```python
from build123d import *

# Parameters (mm, degrees)
SKETCH2_W            = 260
SKETCH2_H            = 260
BOSS_EXTRUDE1_DEPTH  = 500
SKETCH4_W            = 40
SKETCH4_H            = 60
CUT_EXTRUDE1_DEPTH   = 621.644825967
CUT_EXTRUDE2_REACH   = 622.645
MIRROR2_COPY_1_REACH = 622.645


with BuildPart() as part:
    # Sketch2 → Boss-Extrude1 (new body)
    with BuildSketch(Plane(origin=(0, 0, 0), x_dir=(1, 0, 0), z_dir=(0, 1, 0))):
        with Locations((130, 130)):
            Rectangle(SKETCH2_W, SKETCH2_H)
    extrude(amount=BOSS_EXTRUDE1_DEPTH)

    # Sketch4 → Cut-Extrude1 (cut, symmetric)
    with BuildSketch(Plane(origin=(260, 0, 0), x_dir=(0, 0, -1), z_dir=(1, 0, 0))):
        with Locations((20, 370)):
            Rectangle(SKETCH4_W, SKETCH4_H)
    cut_extrude1 = extrude(amount=CUT_EXTRUDE1_DEPTH, both=True, mode=Mode.SUBTRACT)

    # Sketch5 → Cut-Extrude2 (cut, up to next)
    with BuildSketch(Plane(origin=(0, 500, 0), x_dir=(1, 0, 0), z_dir=(0, 1, 0)), mode=Mode.PRIVATE) as cut_extrude2_sk1:
        with BuildLine():
            ThreePointArc((69.556138468, 20.047965883), (67.212992718, 25.704820132), (61.556138468, 28.047965883))
            Line((61.556138468, 28.047965883), (61.556138468, 20.047965883))
            Line((61.556138468, 20.047965883), (61.556138468, 12.047965883))
            ThreePointArc((61.556138468, 12.047965883), (67.212992718, 14.391111633), (69.556138468, 20.047965883))
        make_face()
    cut_extrude2_tool1 = extrude(cut_extrude2_sk1.sketch, amount=-CUT_EXTRUDE2_REACH, mode=Mode.PRIVATE) & part.part
    # Sketch5 → Cut-Extrude2 (cut, up to next)
    with BuildSketch(Plane(origin=(0, 500, 0), x_dir=(1, 0, 0), z_dir=(0, 1, 0)), mode=Mode.PRIVATE) as cut_extrude2_sk2:
        with BuildLine():
            Line((61.556138468, 20.047965883), (61.556138468, 28.047965883))
            ThreePointArc((61.556138468, 28.047965883), (53.556138468, 20.047965883), (61.556138468, 12.047965883))
            Line((61.556138468, 12.047965883), (61.556138468, 20.047965883))
        make_face()
    cut_extrude2_tool2 = extrude(cut_extrude2_sk2.sketch, amount=-CUT_EXTRUDE2_REACH, mode=Mode.PRIVATE) & part.part
    # Sketch5 → Cut-Extrude2 (cut, up to next)
    with BuildSketch(Plane(origin=(0, 500, 0), x_dir=(1, 0, 0), z_dir=(0, 1, 0)), mode=Mode.PRIVATE) as cut_extrude2_sk3:
        with BuildLine():
            ThreePointArc((69.556138468, 20.047965883), (67.212992718, 25.704820132), (61.556138468, 28.047965883))
            Line((61.556138468, 28.047965883), (61.556138468, 20.047965883))
            Line((61.556138468, 20.047965883), (61.556138468, 12.047965883))
            ThreePointArc((61.556138468, 12.047965883), (67.212992718, 14.391111633), (69.556138468, 20.047965883))
        make_face()
    cut_extrude2_tool3 = extrude(cut_extrude2_sk3.sketch, amount=-CUT_EXTRUDE2_REACH, mode=Mode.PRIVATE) & part.part
    # Sketch5 → Cut-Extrude2 (cut, up to next)
    with BuildSketch(Plane(origin=(0, 500, 0), x_dir=(1, 0, 0), z_dir=(0, 1, 0)), mode=Mode.PRIVATE) as cut_extrude2_sk4:
        with BuildLine():
            Line((61.556138468, 20.047965883), (61.556138468, 28.047965883))
            ThreePointArc((61.556138468, 28.047965883), (53.556138468, 20.047965883), (61.556138468, 12.047965883))
            Line((61.556138468, 12.047965883), (61.556138468, 20.047965883))
        make_face()
    cut_extrude2_tool4 = extrude(cut_extrude2_sk4.sketch, amount=-CUT_EXTRUDE2_REACH, mode=Mode.PRIVATE) & part.part
    cut_extrude2_1 = cut_extrude2_tool1.solids().sort_by_distance((64.951444, 500, -20.047966))[0]
    add(cut_extrude2_1, mode=Mode.SUBTRACT)
    cut_extrude2_2 = cut_extrude2_tool2.solids().sort_by_distance((58.160833, 500, -20.047966))[0]
    add(cut_extrude2_2, mode=Mode.SUBTRACT)
    cut_extrude2_3 = cut_extrude2_tool3.solids().sort_by_distance((64.951444, 500, -20.047966))[0]
    add(cut_extrude2_3, mode=Mode.SUBTRACT)
    cut_extrude2_4 = cut_extrude2_tool4.solids().sort_by_distance((58.160833, 500, -20.047966))[0]
    add(cut_extrude2_4, mode=Mode.SUBTRACT)
    cut_extrude2 = cut_extrude2_1 + cut_extrude2_2 + cut_extrude2_3 + cut_extrude2_4  # Cut-Extrude2 as one shape, for the pattern or mirror that repeats it

    # Mirror1: Cut-Extrude2 across plane
    add(cut_extrude2.mirror(Plane.ZY.offset(-130)), mode=Mode.SUBTRACT)

    # Mirror2: Cut-Extrude1, Cut-Extrude2 across plane
    add(cut_extrude1.mirror(Plane(origin=(0, 0, -130), x_dir=(1, 0, 0), z_dir=(0, 0, -1))), mode=Mode.SUBTRACT)
    add(cut_extrude2.mirror(Plane(origin=(0, 0, -130), x_dir=(1, 0, 0), z_dir=(0, 0, -1))), mode=Mode.SUBTRACT)

    # Mirror2 copy 1 sketch → Mirror2 copy 1 (cut, up to next)
    with BuildSketch(Plane(origin=(260, 500, -260), x_dir=(-1, 0, 0), z_dir=(0, 1, 0)), mode=Mode.PRIVATE) as mirror2_copy_1_sk1:
        with BuildLine():
            ThreePointArc((69.556138468, 20.047965883), (67.212992718, 25.704820132), (61.556138468, 28.047965883))
            Line((61.556138468, 28.047965883), (61.556138468, 20.047965883))
            Line((61.556138468, 20.047965883), (61.556138468, 12.047965883))
            ThreePointArc((61.556138468, 12.047965883), (67.212992718, 14.391111633), (69.556138468, 20.047965883))
        make_face()
    mirror2_copy_1_tool1 = extrude(mirror2_copy_1_sk1.sketch, amount=-MIRROR2_COPY_1_REACH, mode=Mode.PRIVATE) & part.part
    # Mirror2 copy 1 sketch → Mirror2 copy 1 (cut, up to next)
    with BuildSketch(Plane(origin=(260, 500, -260), x_dir=(-1, 0, 0), z_dir=(0, 1, 0)), mode=Mode.PRIVATE) as mirror2_copy_1_sk2:
        with BuildLine():
            Line((61.556138468, 20.047965883), (61.556138468, 28.047965883))
            ThreePointArc((61.556138468, 28.047965883), (53.556138468, 20.047965883), (61.556138468, 12.047965883))
            Line((61.556138468, 12.047965883), (61.556138468, 20.047965883))
        make_face()
    mirror2_copy_1_tool2 = extrude(mirror2_copy_1_sk2.sketch, amount=-MIRROR2_COPY_1_REACH, mode=Mode.PRIVATE) & part.part
    # Mirror2 copy 1 sketch → Mirror2 copy 1 (cut, up to next)
    with BuildSketch(Plane(origin=(260, 500, -260), x_dir=(-1, 0, 0), z_dir=(0, 1, 0)), mode=Mode.PRIVATE) as mirror2_copy_1_sk3:
        with BuildLine():
            ThreePointArc((69.556138468, 20.047965883), (67.212992718, 25.704820132), (61.556138468, 28.047965883))
            Line((61.556138468, 28.047965883), (61.556138468, 20.047965883))
            Line((61.556138468, 20.047965883), (61.556138468, 12.047965883))
            ThreePointArc((61.556138468, 12.047965883), (67.212992718, 14.391111633), (69.556138468, 20.047965883))
        make_face()
    mirror2_copy_1_tool3 = extrude(mirror2_copy_1_sk3.sketch, amount=-MIRROR2_COPY_1_REACH, mode=Mode.PRIVATE) & part.part
    # Mirror2 copy 1 sketch → Mirror2 copy 1 (cut, up to next)
    with BuildSketch(Plane(origin=(260, 500, -260), x_dir=(-1, 0, 0), z_dir=(0, 1, 0)), mode=Mode.PRIVATE) as mirror2_copy_1_sk4:
        with BuildLine():
            Line((61.556138468, 20.047965883), (61.556138468, 28.047965883))
            ThreePointArc((61.556138468, 28.047965883), (53.556138468, 20.047965883), (61.556138468, 12.047965883))
            Line((61.556138468, 12.047965883), (61.556138468, 20.047965883))
        make_face()
    mirror2_copy_1_tool4 = extrude(mirror2_copy_1_sk4.sketch, amount=-MIRROR2_COPY_1_REACH, mode=Mode.PRIVATE) & part.part
    add(mirror2_copy_1_tool1.solids().sort_by_distance((195.048556, 500, -239.952034))[0], mode=Mode.SUBTRACT)
    add(mirror2_copy_1_tool2.solids().sort_by_distance((201.839167, 500, -239.952034))[0], mode=Mode.SUBTRACT)
    add(mirror2_copy_1_tool3.solids().sort_by_distance((195.048556, 500, -239.952034))[0], mode=Mode.SUBTRACT)
    add(mirror2_copy_1_tool4.solids().sort_by_distance((201.839167, 500, -239.952034))[0], mode=Mode.SUBTRACT)


solid = part.part
```
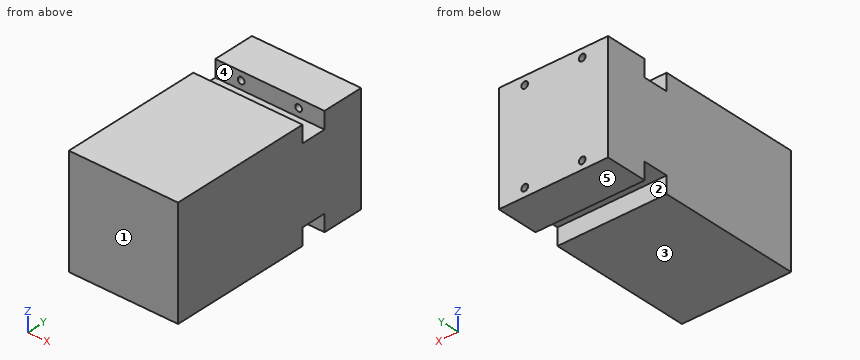
Could you check a few things on this model? Use its own coordinates, in mm. Face numbers are marked on the shaded views. A direction names the side the tool comes from. Give positions to 0.01 mm unless a question says otherwise; leave off trailing zeros. Order: outer loops, then holes, each group sorted by start corner. A loop starts at its lowest first (then second) coordinate and runs counter-clockwise, first axis right, second up.
Q1. Suppose I cut it at A-A, the plane x = 116. Write out the boundary of the cut face in (y, z), and give its area (3 significant figures).
Q2. Suppose I cut it at B-B, the plane y = 358.5. Write out the boundary of the cut face in (x, z), and give its area (3 significant figures).
Q3. If I drill on line 1 along Y through (x, z) = (60, -224.5); line 2 along Z through (x, y) = (112, 398.5), over which ranges is the centre line in solid material (lowest first)?
Q4. We'd pull the mould along Y, two halves only. Please class the marked faces 1, 2 and 3: +Y half, -Y half, draft (parallel to the pull), parting line (faces both ways), or undercut.
Q5. For the marked faces 4 and 5, which set-ups out of +Z, -Z, +X, -X, +Y, -Y let a thin tool reach every point of the face, with its end or its side?
Solution:
1. outline: (0, -260) - (340, -260) - (340, -220) - (400, -220) - (400, -260) - (500, -260) - (500, 0) - (400, 0) - (400, -40) - (340, -40) - (340, 0) - (0, 0) - close
1. area: 125,000 mm2
2. outline: (0, -220) - (260, -220) - (260, -40) - (0, -40) - close
2. area: 46,800 mm2
3. line 1: y = 0 to 340, 400 to 500
3. line 2: z = -220 to -40
4. face 1: -Y half
4. face 2: undercut
4. face 3: draft
5. face 4: +Z, +X, -X
5. face 5: -Z, +X, -X, +Y, -Y
